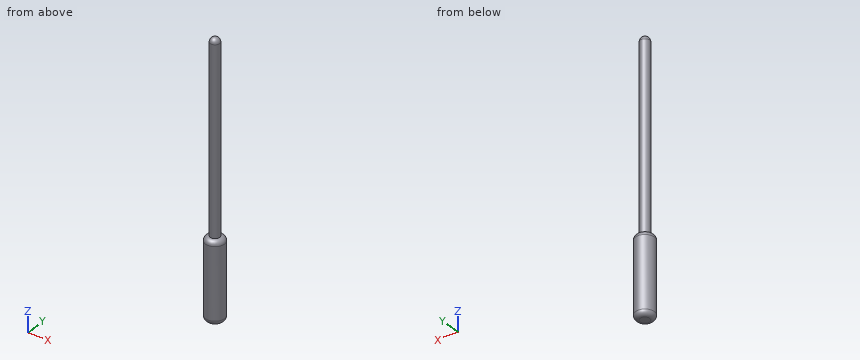
from build123d import *

# Parameters (mm, degrees)
F0_R     = 5
F1_DEPTH = 200
F2_R     = 10
F2_R_2   = 5
F3_DEPTH = 85
F4_R     = 4.99999
F5_R     = 5


# Not quite as in the source:
# - a fillet or chamfer is up to 0.001 mm smaller than in the source, because OpenCascade refuses the exact size


with BuildPart() as f1:
    # F0 (on Top) → F1 (new body)
    with BuildSketch(Plane.XY):
        Circle(F0_R)
    extrude(amount=F1_DEPTH)

    # F2 (on face) → F3 (join)
    with BuildSketch(Plane(origin=(0, 0, 0), x_dir=(1, 0, 0), z_dir=(0, 0, -1))):
        Circle(F2_R)
        Circle(F2_R_2, mode=Mode.SUBTRACT)
        Circle(F2_R_2)
    extrude(amount=F3_DEPTH)

    # F4 (radius 5 in the source; OpenCascade refuses exactly that, so slightly less here)
    f4_edges = [f1.edges().sort_by_distance(p)[0] for p in [
        (-10, 0, 0),
        (-10, 0, -85),
    ]]
    fillet(f4_edges, radius=F4_R)

    # F5
    f5_edges = [f1.edges().sort_by_distance(p)[0] for p in [
        (-5, 0, 200),
    ]]
    fillet(f5_edges, radius=F5_R)


solid = f1.part
Check sheet for the modelled part. Datum: model origin and axes. Units: mm. Give positions to 0.01 mm unless a question says otherwise; leave off trailing zeros. Loops run counter-clockwise (first coordinate to the right, second up) from the corner with the lowest first, then second, coordinate; pieces in that order, holes last. Notation, with made-up numbers: M 6.5,-11.75 L 17.5,-11.75 A10 cw 17.5,-7.75 Z; hole C -21,-17.75 d6. An arc over 180 degrees is marked long. Return JSON: item names as keys, results as strings. Group by question number.
1. Cross-section at C-C on z = 97. Record the boundary of the cut face in (x, y), plus the area to 3 significant figures.
2. Go/stop test with flat-tipped pins: pin 1 (4 mm diameter, centred on x = 0.5, y = 6, fed in from +Z); pin 2 (3 mm diameter, centred on y = 2, z = 70.5, fed in from -X); pin 3 (4 mm diameter, centred on y = 5.5, z = -38, fed in from +X). Record where each tip stops, or that it passes through.
3. Cross-section at D-D on z = -35. Record the boundary of the cut face in (x, y).
4. Thickness scan on L1, parallel to Y at x = -0.25, z = 66; L2, parallel to Z at x = 5, y = 2; L3, parallel to X at y = -2.5, z = 28.5. Record the ranges inside material, lowest first.
Return value:
{
 "1": {"outline": "C 0,0 d10", "area": "78.5 mm^2"},
 "2": {"pin 1": "z = 197.97", "pin 2": "x = -4.97", "pin 3": "x = 9.37"},
 "3": {"outline": "C 0,0 d20"},
 "4": {"L1": "-4.99 to 4.99", "L2": "-84.99 to -0.01", "L3": "-4.33 to 4.33"}
}
